Job drawing, mm, ordinate dimensions from the low corner. One solid piece. A direction names the side the tool comes from. Coordinates: 2 decimals unless noted, no trailing zeros. Order: outer loops, then holes, each group sorted by start corner. A loop starts at its lowest first (then second) coordinate and runs counter-clockwise, first axis right, second up. Notation, with made-up numbers: (83.5, 76.25) - (138.5, 76.25) arc R23 cw to (138.5, 109.25) - close; hole circle Ø9 at (5, 85.5). An arc over 180 degrees is marked (long way). Return JSON: item names as keys, results as strings.
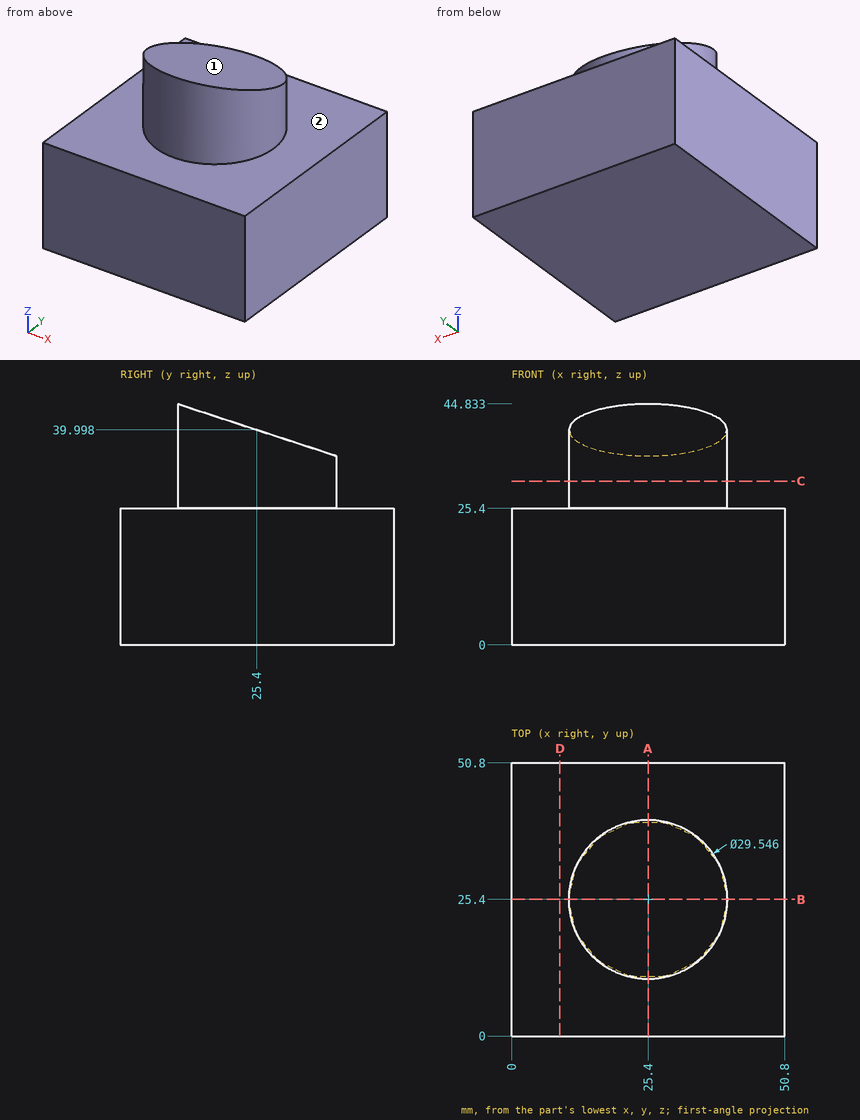
1. Cut at D-D on x = 9. Give the cut face in (y, z).
Check values:
{"outline": "(0, 0) - (50.8, 0) - (50.8, 25.4) - (0, 25.4) - close"}
2. Tool access for the marked faces 1 and 2: list every direction of +Z, -Z, +X, -X, +Y, -Y with a clear straight run to the whole face (end or side of a thin tool).
Check values:
{"face 1": "+Z, +X, -X, +Y", "face 2": "+Z"}
3. Cut at C-C on z = 30.5. Give the cut face in (x, y).
Check values:
{"outline": "circle Ø29.55 at (25.4, 25.4)"}
4. Probe L1, parallel to Z at x = 3, y = 23; L2, parallel to Z at x = 27.5, y = 21.5 (1 decimal); L3, parallel to X at y = 26.5, z = 34. List the from-to ranges inside material, lowest first.
Check values:
{"L1": "0 to 25.4", "L2": "0 to 41.3", "L3": "10.67 to 40.13"}
5. Cut at A-A on x = 25.4. Give the cut face in (y, z), plus the area to 3 significant figures.
Check values:
{"outline": "(0, 0) - (50.8, 0) - (50.8, 25.4) - (40.17, 25.4) - (40.17, 35.16) - (10.63, 44.83) - (10.63, 25.4) - (0, 25.4) - close", "area": "1,720 mm²"}
6. Cut at B-B on y = 25.4. Give the cut face in (x, z).
Check values:
{"outline": "(0, 0) - (50.8, 0) - (50.8, 25.4) - (40.17, 25.4) - (40.17, 40) - (10.63, 40) - (10.63, 25.4) - (0, 25.4) - close"}
7. Drop flat-ended pins along their axis: pin 1 (1.5 mm diameter, centred on x = 44, y = 42, fed in from +Z); pin 2 (3 mm diameter, centred on x = 29, y = 38, fed in from +Z) (1 decimal); pin 3 (5 mm diameter, centred on x = 39.5, y = 34, fed in from +Z). Give the stop position or say it passes through.
Check values:
{"pin 1": "z = 25.4", "pin 2": "z = 36.4", "pin 3": "z = 37.97"}
